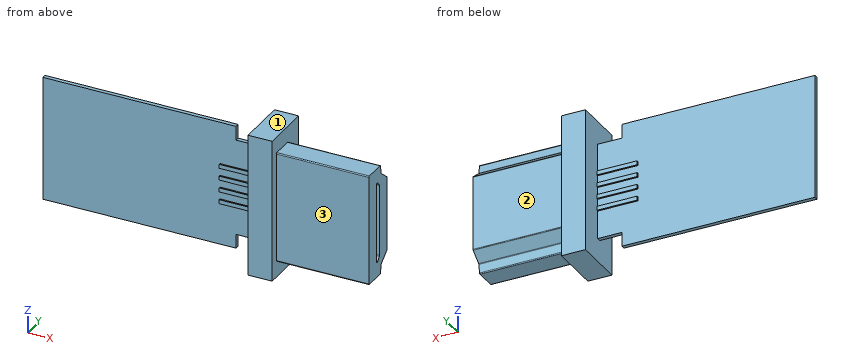
from build123d import *

# Parameters (mm, degrees)
BOSS_EXTRUDE1_DEPTH = 11.5
SKETCH2_W           = 17.8
SKETCH2_H           = 6.4
BOSS_EXTRUDE2_DEPTH = 3
BOSS_EXTRUDE3_DEPTH = 0.25
SKETCH4_W           = 5
SKETCH4_H           = 0.5
BOSS_EXTRUDE4_DEPTH = 0.2
FILLET1_R           = 0.125
CUT_EXTRUDE1_DEPTH  = 6.5
FILLET2_R           = 0.2


with BuildPart() as part:
    # Sketch1 → Boss-Extrude1 (new body)
    with BuildSketch(Plane(origin=(0, 0, 0), x_dir=(0, 0, -1), z_dir=(1, 0, 0))):
        Polygon((0, 2.8), (1.152683079, 3.000553531), (2.25, 4.4), (11.55, 4.4), (12.647316921, 3.000553531), (13.8, 2.8), (13.8, 0), (0, 0), align=None)
    extrude(amount=BOSS_EXTRUDE1_DEPTH)

    # Sketch2 → Boss-Extrude2 (add)
    with BuildSketch(Plane.ZY):
        with Locations((-6.9, 2.2)):
            Rectangle(SKETCH2_W, SKETCH2_H)
    extrude(amount=BOSS_EXTRUDE2_DEPTH)

    # Sketch3 → Boss-Extrude3 (add, symmetric)
    with BuildSketch(Plane(origin=(0, 2.2, 0), x_dir=(1, 0, 0), z_dir=(0, 1, 0))):
        Polygon((-3, 12.9), (-6, 12.9), (-6, 14.65), (-30, 14.65), (-30, -0.85), (-6, -0.85), (-6, 0.9), (-3, 0.9), align=None)
    extrude(amount=BOSS_EXTRUDE3_DEPTH, both=True)

    # Sketch4 → Boss-Extrude4 (add)
    with BuildSketch(Plane(origin=(0, 2.45, 0), x_dir=(1, 0, 0), z_dir=(0, 1, 0))):
        with Locations((-5.5, 9.15)):
            Rectangle(SKETCH4_W, SKETCH4_H)
        with Locations((-5.5, 7.65)):
            Rectangle(SKETCH4_W, SKETCH4_H)
        with Locations((-5.5, 6.15)):
            Rectangle(SKETCH4_W, SKETCH4_H)
        with Locations((-5.5, 4.65)):
            Rectangle(SKETCH4_W, SKETCH4_H)
    boss_extrude4 = extrude(amount=BOSS_EXTRUDE4_DEPTH)

    # Mirror1: Boss-Extrude4 across plane
    add(boss_extrude4.mirror(Plane.ZX.offset(2.2)))

    # Fillet1
    fillet1_edges = [part.edges().sort_by_distance(p)[0] for p in [
        (5.75, 2.8, 0),
        (5.75, 3.000553531, -1.152683079),
        (5.75, 4.4, -2.25),
        (5.75, 4.4, -11.55),
        (5.75, 3.000553531, -12.647316921),
        (5.75, 2.8, -13.8),
        (5.75, 0, -13.8),
        (5.75, 0, 0),
    ]]
    fillet(fillet1_edges, radius=FILLET1_R)

    # Sketch5 → Cut-Extrude1 (cut)
    with BuildSketch(Plane(origin=(11.5, 0, 0), x_dir=(0, 0, -1), z_dir=(1, 0, 0))):
        Polygon((2.4, 2.5825), (1.5, 1.8175), (12.3, 1.8175), (11.4, 2.5825), align=None)
    extrude(amount=-CUT_EXTRUDE1_DEPTH, mode=Mode.SUBTRACT)

    # Fillet2
    fillet2_edges = [part.edges().sort_by_distance(p)[0] for p in [
        (8.25, 1.8175, -1.5),
        (8.25, 1.8175, -12.3),
        (8.25, 2.5825, -11.4),
        (8.25, 2.5825, -2.4),
    ]]
    fillet(fillet2_edges, radius=FILLET2_R)


solid = part.part
Can you work these out from the model? Positions are in its coordinate system, mm. Face numbers are marked on the shaded views. A direction names the side the tool comes from. Give positions to 0.01 mm unless a question says otherwise; leave off trailing zeros. Write each loop counter-clockwise with the first axis right and the second up, starting at its lowest first coordinate (ties: lowest second). Pieces come first, ordered by that corner, then holes. Notation, with made-up numbers: (72.25, 73) -> (102.25, 73) arc R27 cw to (102.25, 106) -> close; hole circle Ø6 at (72, -33). An arc over 180 degrees is marked (long way). Answer as a JSON object with one key per item and string values. Group by question number.
Item 1: Please list where these lines run through material, in increasing order: line 1 (X direction, y = 3.75, z = -13.5); line 2 (X direction, y = 2, z = -6.25); line 3 (Y direction, x = -3.5, z = -9.75). Write a range as [from, to].
Item 2: Suppose I cut it at A-A (z = -14.25). Please give me the cut outline in (x, y).
Item 3: Suppose I cut it at D-D (z = -8.5). Please give me the cut outline in (x, y).
Item 4: For the marked faces 1, 2 and 3, which set-ups out of +Z, -Z, +X, -X, +Y, -Y let a thin tool reach every point of the face, with its end or its side?
Item 5: Suppose I cut it at C-C (y = 1). Please give me the cut outline in (x, z).
Item 6: I'm going to push flat-ended pins straight in: P1, Ø3, axis at x = -19.5, z = -12, coming from the +Y side; P2, Ø7, axis at x = 7.5, z = -7, coming from the +Y side; P3, Ø7, axis at x = 10, z = -6, coming from the -Y side; P4, Ø1.5, axis at x = -19, y = 3.5, coming from the -Z side. Where does each tip first touch, or does it pass through?
Findings:
{
 "1": {"line 1": "x = [-3, 0]", "line 2": "x = [-30, 5]", "line 3": "y = [1.95, 2.45]"},
 "2": {"outline": "(-30, 1.95) -> (-6, 1.95) -> (-6, 2.45) -> (-30, 2.45) -> close; (-3, -1) -> (0, -1) -> (0, 5.4) -> (-3, 5.4) -> close"},
 "3": {"outline": "(-30, 1.95) -> (-3, 1.95) -> (-3, -1) -> (0, -1) -> (0, 0) -> (11.5, 0) -> (11.5, 1.82) -> (5, 1.82) -> (5, 2.58) -> (11.5, 2.58) -> (11.5, 4.4) -> (0, 4.4) -> (0, 5.4) -> (-3, 5.4) -> (-3, 2.45) -> (-30, 2.45) -> close"},
 "4": {"face 1": "+Z, +X, -X, +Y, -Y", "face 2": "+Z, -Z, +X, +Y", "face 3": "+Z, -Z, +X, -Y"},
 "5": {"outline": "(-3, -15.8) -> (0, -15.8) -> (0, -13.8) -> (11.5, -13.8) -> (11.5, 0) -> (0, 0) -> (0, 2) -> (-3, 2) -> close"},
 "6": {"P1": "stops at y = 2.45", "P2": "stops at y = 4.4", "P3": "stops at y = 0", "P4": "passes through"}
}
